Check sheet for the modelled part. Datum: model origin and axes. Units: mm. Give positions to 0.01 mm unless a question says otherwise; leave off trailing zeros. Order: outer loops, then holes, each group sorted by start corner. A loop starts at its lowest first (then second) coordinate and runs counter-clockwise, first axis right, second up.
```python
from build123d import *

# Parameters (mm, degrees)
BOSS_EXTRUDE1_DEPTH = 3.5
BOSS_EXTRUDE3_DEPTH = 4
SKETCH4_R           = 1.25
CUT_EXTRUDE1_DEPTH  = 4


with BuildPart() as part:
    # Sketch1 → Boss-Extrude1 (new body)
    with BuildSketch(Plane(origin=(0, 0, 0), x_dir=(0, 0, -1), z_dir=(1, 0, 0))):
        Polygon((0, 30.375), (25, 30.375), (25, 9.375), (21.5, 9.375), (21.5, 26.875), (0, 26.875), align=None)
    extrude(amount=BOSS_EXTRUDE1_DEPTH)

    # Sketch3 → Boss-Extrude3 (add)
    with BuildSketch(Plane(origin=(0, 9.375, 0), x_dir=(-1, 0, 0), z_dir=(0, -1, 0))):
        with BuildLine():
            Line((4.554760106, 24.5), (4.003093597, 21.04375))
            ThreePointArc((4.003093597, 21.04375), (-1.75, 21.5), (-7.503093597, 21.04375))
            Line((-7.503093597, 21.04375), (-8.054760106, 24.5))
            ThreePointArc((-8.054760106, 24.5), (-1.75, 25), (4.554760106, 24.5))
        make_face()
    extrude(amount=-BOSS_EXTRUDE3_DEPTH)

    # Sketch4 → Cut-Extrude1 (cut)
    with BuildSketch(Plane(origin=(0, 30.375, 0), x_dir=(1, 0, 0), z_dir=(0, 1, 0))):
        with Locations(Location((1.75, 1.75, 0), (0, 0, 270))):
            Circle(SKETCH4_R)
    extrude(amount=-CUT_EXTRUDE1_DEPTH, mode=Mode.SUBTRACT)


solid = part.part
```
(1) Cross-section at A-A on z = -1.75. Enter the section's corners in (x, y) (3 decimals), then the cut area to 3 significant figures.
Response values:
outline: (0, 26.875) - (0.5, 26.875) - (0.5, 30.375) - (0, 30.375) - close; (3, 26.875) - (3.5, 26.875) - (3.5, 30.375) - (3, 30.375) - close
area: 3.50 mm2
(2) Cross-section at D-D on y = 18.25. Enter the section's corners in (x, z).
Response values:
outline: (0, -25) - (3.5, -25) - (3.5, -21.5) - (0, -21.5) - close
(3) Release check for a two-part mould opening along Y. For faces 1 (the face through (2, 30.375, -12)), 2 (the face through (1.7, 11.3, -21.5)), 3 (the face through (2, 20, -21.5)) record: released by +Y, released by -Y, zero draft, split by the parting line, or undercut.
Response values:
face 1: released by +Y
face 2: zero draft
face 3: undercut
(4) Cross-section at B-B on x = 2.5. Enter the section's corners in (y, z) (3 decimals).
Response values:
outline: (9.375, -25) - (30.375, -25) - (30.375, -2.75) - (26.875, -2.75) - (26.875, -21.5) - (13.375, -21.5) - (13.375, -21.492) - (9.375, -21.492) - close; (26.875, -0.75) - (30.375, -0.75) - (30.375, 0) - (26.875, 0) - close
(5) Gauge pin test, flat ends, axial feed: pin 1 Ø2 at (x, z) = (-3, -22) entering from +Y (3 decimals); pin 2 Ø3 at (x, y) = (-2.5, 23.5) entering from +Z; pin 3 Ø3 at (x, y) = (1, 21.5) entering from +Z; pin 4 Ø10.5 at (y, z) = (23, -14.5) entering from -X. Record the tip position at first contact, or that the pin passes through.
Response values:
pin 1: stops at y = 13.375
pin 2: passes through
pin 3: stops at z = -21.5
pin 4: stops at x = 0
(6) Cross-section at C-C on z = -11. Enter the section's corners in (x, y) (3 decimals), then the cut area to 4 significant figures.
Response values:
outline: (0, 26.875) - (3.5, 26.875) - (3.5, 30.375) - (0, 30.375) - close
area: 12.25 mm2
(7) Material ranges on L1, parallel to X at y = 28.8, z = -1.75; L2, parallel to Y at x = 2.75, z = -5 (3 decimals); L3, parallel to Z at x = 3.25, y = 26.5, recorded low to high.
Response values:
L1: x = 0 to 0.5, 3 to 3.5
L2: y = 26.875 to 30.375
L3: z = -25 to -21.5
